```python
from build123d import *

# Parameters (mm, degrees)
F0_W     = 79.085034
F0_H     = 93.884569
F1_DEPTH = 50.038
F2_W     = 62.076326
F2_H     = 23.337272
F3_DEPTH = 124.46
F4_W     = 71.68526
F4_H     = 86.253557
F5_DEPTH = 46.736
F6_R     = 9.296837
F7_DEPTH = 141.986


with BuildPart() as f1:
    # F0 (on Top) → F1 (new body)
    with BuildSketch(Plane.XY):
        with Locations((5.318584, -0.231241)):
            Rectangle(F0_W, F0_H)
    extrude(amount=F1_DEPTH)

    # F2 (on face) → F3 (cut)
    with BuildSketch(Plane(origin=(-34.223933, 0, 0), x_dir=(0, -1, 0), z_dir=(-1, 0, 0))):
        with Locations((0.123933, 38.369364)):
            Rectangle(F2_W, F2_H)
    extrude(amount=-F3_DEPTH, mode=Mode.SUBTRACT)

    # F4 (on face) → F5 (cut)
    with BuildSketch(Plane.XY.offset(50.038)):
        with Locations((5.318583, -0.346864)):
            Rectangle(F4_W, F4_H)
    extrude(amount=-F5_DEPTH, mode=Mode.SUBTRACT)

    # F6 (on face) → F7 (cut)
    with BuildSketch(Plane.XZ.offset(47.173526)):
        with Locations((4.334087, 24.607167)):
            Circle(F6_R)
    extrude(amount=-F7_DEPTH, mode=Mode.SUBTRACT)


solid = f1.part
```
Source: CAD feature listing. Evaluate the final solid. Frame: model axes, mm. A direction names the side the tool comes from. Give positions to 0.01 mm unless a question says otherwise; leave off trailing zeros. Loops run counter-clockwise (first coordinate to the right, second up) from the corner with the lowest first, then second, coordinate; pieces in that order, holes last. Notation, with made-up numbers: (27.25, 54) - (37.25, 54) arc R35 ccw to (37.25, 88) - close; hole circle Ø7 at (-28, 55). An arc over 180 degrees is marked (long way). Use CSV: the item, a comma, the result in double quotes. Start each with the question number.
1. Pin query (flat end, axial travel): pin 1 (4 mm diameter, centred on x = -32.5, y = 5, fed in from +Z). Return the tip coordinate at first contact, or that it passes through.
2. Draft query along X for faces 1 (the flat face through (5, 0, 3.302)), 2 (the flat face through (41.161, -1, 17)), 3 (the flat face through (-32, -31.162, 38)), 4 (the flat face through (44.861, -1, 19)). Return one class per face: +X half, -X half, draft (parallel to the pull), parting line (faces both ways), or undercut.
3. Section C-C (z = 44). Output: boundary loops of the cut face in (x, y), then the cut area to 3 significant figures.
4. Section B-B (y = 29). Output: boundary loops of the cut face in (x, z), then the cut area to 3 significant figures.
5. Section A-A (z = 8). Output: boundary loops of the cut face in (x, y), then the cut area to 3 significant figures.
6. Reachability of faces 5 (the cylindrical face through (9.332, -45.349, 32.446)), 6 (the flat face through (43, 0, 26.701)), 7 (the flat face through (-3, -43.474, 32)) from +Z, -Z, +X, -X, +Y, -Y: full face, straight path, thin tool, end or side. Return the list, or none.
7. Section D-D (x = -22). Output: boundary loops of the cut face in (y, z), then the cut area to 3 significant figures.
8. Ray query, L1, parallel to Y at x = 35, z = 26.5; L2, parallel to X at y = -19, z = 10.5; L3, parallel to Z at x = -29, y = -7.5. Return the intervals inside material, ascending.
Response:
1,pin 1,"z = 26.7"
2,face 1,"undercut"
2,face 2,"undercut"
2,face 3,"draft"
2,face 4,"+X half"
3,outline,"(-34.22, -47.17) - (44.86, -47.17) - (44.86, -31.16) - (41.16, -31.16) - (41.16, -43.47) - (-30.52, -43.47) - (-30.52, -31.16) - (-34.22, -31.16) - close; (-34.22, 30.91) - (-30.52, 30.91) - (-30.52, 42.78) - (41.16, 42.78) - (41.16, 30.91) - (44.86, 30.91) - (44.86, 46.71) - (-34.22, 46.71) - close"
3,area,"782 mm²"
4,outline,"(-34.22, 0) - (44.86, 0) - (44.86, 26.7) - (41.16, 26.7) - (41.16, 3.3) - (-30.52, 3.3) - (-30.52, 26.7) - (-34.22, 26.7) - close"
4,area,"434 mm²"
5,outline,"(-34.22, -47.17) - (44.86, -47.17) - (44.86, 46.71) - (-34.22, 46.71) - close; hole (-30.52, -43.47) - (41.16, -43.47) - (41.16, 42.78) - (-30.52, 42.78) - close"
5,area,"1,240 mm²"
6,face 5,"+Y, -Y"
6,face 6,"+Z, +X, -X"
6,face 7,"+Z"
7,outline,"(-47.17, 0) - (46.71, 0) - (46.71, 50.04) - (42.78, 50.04) - (42.78, 3.3) - (-43.47, 3.3) - (-43.47, 50.04) - (-47.17, 50.04) - close"
7,area,"667 mm²"
8,L1,"-47.17 to -43.47, 42.78 to 46.71"
8,L2,"-34.22 to -30.52, 41.16 to 44.86"
8,L3,"0 to 3.3"
